```python
from build123d import *

# Parameters (mm, degrees)
F0_R     = 9.575
F0_R_2   = 11.025
F1_DEPTH = 3.5


# Not quite as in the source:
# - a feature names something its author has since deleted; it is built from what else it names


with BuildPart() as f1:
    # F0 (on Top) → F1 (new body, symmetric)
    with BuildSketch(Plane.XY):
        with BuildLine():
            ThreePointArc((-9.7584878157, 25.4313524375), (-10.5871605613, 6.1125), (-26.9034411714, -4.2645778678))
            ThreePointArc((-26.9034411714, -4.2645778678), (-35.3121858393, -20.3875), (-17.1449533556, -21.1667745697))
            ThreePointArc((-17.1449533556, -21.1667745697), (0, -12.225), (17.1449533556, -21.1667745697))
            ThreePointArc((17.1449533556, -21.1667745697), (35.3121858393, -20.3875), (26.9034411714, -4.2645778678))
            ThreePointArc((26.9034411714, -4.2645778678), (10.5871605613, 6.1125), (9.7584878157, 25.4313524375))
            ThreePointArc((9.7584878157, 25.4313524375), (0, 40.775), (-9.7584878157, 25.4313524375))
        make_face()
        with Locations((-25.9807621135, -15)):
            Circle(F0_R, mode=Mode.SUBTRACT)
        Circle(F0_R_2, mode=Mode.SUBTRACT)
        with Locations((25.9807621135, -15)):
            Circle(F0_R, mode=Mode.SUBTRACT)
        with Locations((0, 30)):
            Circle(F0_R, mode=Mode.SUBTRACT)
    extrude(amount=F1_DEPTH, both=True)

    # F4: sweep along a path in F0
    with BuildLine(Plane.XY) as f4_path:
        ThreePointArc((9.7584878157, 25.4313524375), (0, 40.775), (-9.7584878157, 25.4313524375))
    # F3 (on line) → F4 (sweep)
    with BuildSketch(Plane(origin=(11.5201166848, 24.6066077034, 0), x_dir=(-0.9056601221, 0.4240044141, 0), z_dir=(0.4240044141, 0.9056601221, 0))):
        with BuildLine():
            ThreePointArc((1.9451324245, 3.5), (0.9451324245, 0), (1.9451324245, -3.5))
            Line((1.9451324245, -3.5), (1.9451324245, 3.5))
        make_face()
    sweep(path=f4_path.line)

    # F5: sweep along a path in F0
    with BuildLine(Plane.XY) as f5_path:
        ThreePointArc((9.7584878157, 25.4313524375), (10.5871605613, 6.1125), (26.9034411714, -4.2645778678))
        ThreePointArc((26.9034411714, -4.2645778678), (35.3121858393, -20.3875), (17.1449533556, -21.1667745697))
        ThreePointArc((17.1449533556, -21.1667745697), (0, -12.225), (-17.1449533556, -21.1667745697))
        ThreePointArc((-17.1449533556, -21.1667745697), (-35.3121858393, -20.3875), (-26.9034411714, -4.2645778678))
        ThreePointArc((-26.9034411714, -4.2645778678), (-10.5871605613, 6.1125), (-9.7584878157, 25.4313524375))
    # F4_face (on face) → F5 (sweep)
    with BuildSketch(Plane(origin=(10.1232025909, 25.2606033113, 0), x_dir=(0.9056601221, -0.4240044141, 0), z_dir=(-0.4240044141, -0.9056601221, 0))):
        with BuildLine():
            ThreePointArc((-0.402706011, -3.5), (0.597293989, 0), (-0.402706011, 3.5))
            Line((-0.402706011, 3.5), (-0.402706011, -3.5))
        make_face()
    sweep(path=f5_path.line)


solid = f1.part
```
Check sheet for the modelled part. Datum: model origin and axes. Units: mm. Round coordinates to 2 decimals unless told otherwise and drop trailing zeros. Answer as CSV lines item,"result". Start each with the question number.
1) Depth check by flat-ended pin: pin 1 (3 mm diameter, centred on y = 17.5, z = -2.5, fed in from -X); pin 2 (2 mm diameter, centred on y = 19.5, z = -1, fed in from -X). Enter the tip coordinate at first touch or a pass-through.
2) Draft check along Y on faces 1 (the face through (18.92, -8.53, -0.05)), 2 (the face through (-11, -2, 3.5)), 3 (the face through (-2.39, -10.763, -0.049)). Enter one of: +Y half, -Y half, draft (parallel to the pull), parting line (faces both ways), or undercut.
3) Section check A-A (x = 6). Give the number of separate pieces and of enclosed holes in the cut face, then the cut area to 3 significant figures.
4) Scan lines: probe 1 along Y at (x, z) = (0, -1.75) (3 decimals); probe 2 along X at (y, z) = (-21, -0.5); probe 3 along X at (y, z) = (-9.5, -0.25). Record each from-to range of solid material in increasing order.
Determined:
1,pin 1,"x = -8.75"
1,pin 2,"x = -9.13"
2,face 1,"undercut"
2,face 2,"draft"
2,face 3,"undercut"
3,separate pieces,"3"
3,enclosed holes,"0"
3,area,"141 mm^2"
4,probe 1,"-12.99 to -11.025, 11.025 to 20.425, 39.575 to 41.54"
4,probe 2,"-36.09 to -33.44, -18.52 to -15.81, 15.81 to 18.52, 33.44 to 36.09"
4,probe 3,"-36.39 to -33.82, -18.14 to -5.59, 5.59 to 18.14, 33.82 to 36.39"
